Design review of the part shown in the three views and the two pictorial views. Dimensions are in mm from the part's minimum x, y and z. A direction names the side the tool comes from. Coordinates: 2 decimals unless noted, no trailing zeros. Loops run counter-clockwise (first coordinate to the right, second up) from the corner with the lowest first, then second, coordinate; pieces in that order, holes last.
Q1. Wall thickness on probe 1 along X at (y, z) = (14.25, 8.25); probe 2 along X at (y, z) = (23.5, 1); probe 3 along Z at (x, y) = (28.5, 10): over which ranges is each line inside the solid? List them lowest first.
Q2. Add section C-C on z = 1. Give the boundary of the cut face in (x, y) (3 decimals), and give its area (3 significant figures).
Q3. Add section D-D on x = 11. Give the boundary of the cut face in (y, z), and give its area (3 significant figures).
Q4. For P1, Ø0.5, axis at x = 5, z = 0.5, coming from the -Y side; P2, Ø1.7, axis at x = 6, z = 0.5, coming from the +Y side; P3, Ø5, axis at x = 18.5, z = 6.5, coming from the +Y side; P4, Ø2, axis at x = 24.5, y = 19.5, coming from the +Z side, all flat-tipped, find the tip position at first contact; note any pin that passes through.
Q5. Add section B-B on z = 6.75. Give the boundary of the cut face in (x, y) (3 decimals), and give its area (3 significant figures).
Q6. Machinability: for the marked faces 3 and 4, which of the approach directions +Z, -Z, +X, -X, +Y, -Y give a long, thin tool a straight path to every point of the face, cutting with its end or side? Answer none if there is none.
Q7. Add section A-A on y = 25. Give the boundary of the cut face in (x, z).
Q8. Draft analysis for pull direction X (two halves, no side actions). For the marked faces 1 and 2, state which applies: released by +X, released by -X, zero draft, split by the parting line, or undercut.
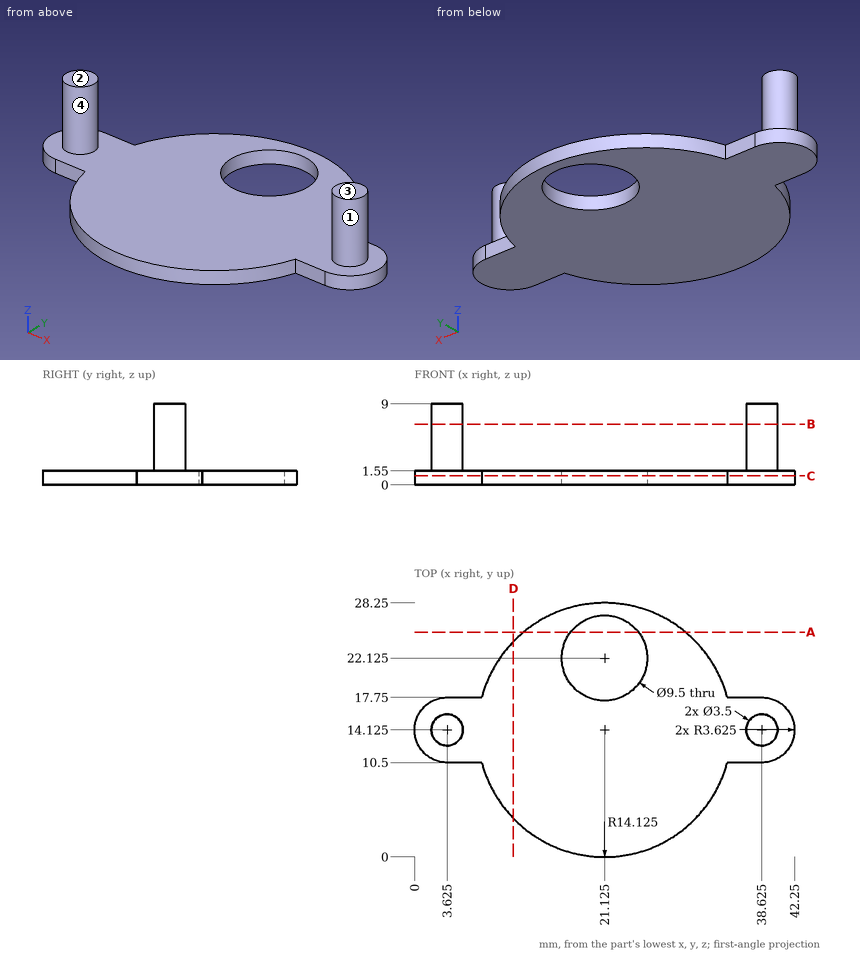
Entries:
1. probe 1: x = 1.88 to 5.37, 36.88 to 40.37
1. probe 2: x = 10.56 to 16.58, 25.67 to 31.69
1. probe 3: z = 0 to 1.55
2. outline: (3.625, 10.5) - (7.473, 10.5) arc R14.125 ccw to (34.777, 10.5) - (38.625, 10.5) arc R3.625 ccw to (38.625, 17.75) - (34.777, 17.75) arc R14.125 ccw to (7.473, 17.75) - (3.625, 17.75) arc R3.625 ccw to start; hole circle Ø9.5 at (21.125, 22.125)
2. area: 648 mm2
3. outline: (4.28, 0) - (23.97, 0) - (23.97, 1.55) - (4.28, 1.55) - close
3. area: 30.5 mm2
4. P1: stops at y = 10.5
4. P2: stops at y = 17.75
4. P3: passes through
4. P4: stops at z = 1.55
5. outline: circle Ø3.5 at (3.625, 14.125); circle Ø3.5 at (38.625, 14.125)
5. area: 19.2 mm2
6. face 3: +Z, +X, -X, +Y, -Y
6. face 4: +Z
7. outline: (12.11, 0) - (17.34, 0) - (17.34, 1.55) - (12.11, 1.55) - close; (24.91, 0) - (30.14, 0) - (30.14, 1.55) - (24.91, 1.55) - close
8. face 1: undercut
8. face 2: zero draft
